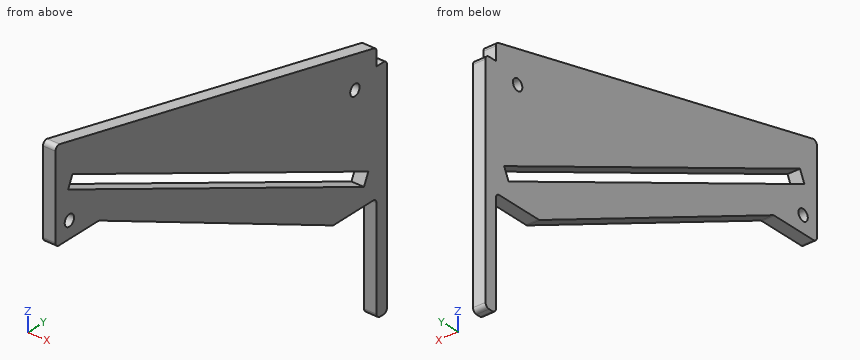
Autodesk Inventor part; units mm, degrees
ref_plane "YZ Plane" through (0, 0, 0) normal (1, 0, 0) x (0, 1, 0)
ref_plane "XZ Plane" through (0, 0, 0) normal (0, 1, 0) x (-1, 0, 0)
ref_plane "XY Plane" through (0, 0, 0) normal (0, 0, 1) x (1, 0, 0)
sketch "Sketch1" plane through (0, 0, 0) normal (1, 0, 0) x (0, 1, 0)
  line L0 (0, 0) -> (0, 25) construction
  line L1 (185, -25) -> (185, -90)
  line L2 (185, -25) -> (-25, 25) construction
  line L3 (0, 0) -> (0, 19.0476)
  line L4 (0, 19.0476) -> (185, -25)
  line L5 (0, -25) -> (0, 0)
  line L6 (185, -90) -> (160, -90)
  line L7 (0, -25) -> (25, -25)
  line L8 (25, -25) -> (160, -90)
  dimension "d0" = 25
  dimension "d1" = 65
  dimension "d2" = 185
  dimension "d10" = 25
  dimension "d11" = 25
  dimension "d17" = 25
  dimension "d20" = 25
extrude "Extrusion1" add sketch "Sketch1" along normal blind 6
sketch "Sketch3" plane through (6, 0, 0) normal (1, 0, 0) x (0, 0, -1)
  line L0 (90, 185) -> (25, 185)
  line L1 (33.1, 185) -> (141.9, 185)
  line L2 (141.9, 185) -> (141.9, 191)
  line L3 (141.9, 191) -> (33.1, 191)
  line L4 (33.1, 191) -> (33.1, 185)
  dimension "d12" = 8.1
  dimension "d14" = 6
  dimension "d21" = 108.8
extrude "Extrusion3" add sketch "Sketch3" against normal blind 6
sketch "Sketch4" plane through (6, 0, 0) normal (1, 0, 0) x (0, 0, -1)
  line L0 (0, 0) -> (85, 185) construction
  line L1 (3.34, 7.2694) -> (-2.1121, 9.7744)
  line L2 (-2.1121, 9.7744) -> (76.2079, 180.2356)
  line L3 (76.2079, 180.2356) -> (81.66, 177.7306)
  line L4 (3.34, 7.2694) -> (81.66, 177.7306)
  dimension "d23" = 185
  dimension "d24" = 85
  dimension "d28" = 8
  dimension "d29" = 8
  dimension "d32" = 6
extrude "Extrusion4" cut sketch "Sketch4" against normal through all
sketch "Sketch5" plane through (6, 0, 0) normal (1, 0, 0) x (0, 0, -1)
  line L0 (-19.0476, 0) -> (25, 0)
  line L1 (25, 0) -> (25, 25)
  line L2 (33.1, 185) -> (25, 185)
  circle A0 centre (37.5, 172.5) radius 2.7
  circle A1 centre (17, 8) radius 2.7
  point P0 (0, 0)
  dimension "d34" = 12.5
  dimension "d35" = 12.5
  dimension "d36" = 5.4
  dimension "d37" = 5.4
  dimension "d38" = 8
  dimension "d39" = 8
extrude "Extrusion5" cut sketch "Sketch5" against normal through all
fillet "Fillet1" radius 2 9 edges at (3, 185, -25) (3, 191, -33.1) (3, 191, -141.9) (3, 185, -141.9) (3, 185, -90) (3, 160, -90) (3, 25, -25) (3, 0, -25) (3, 0, 19.0476)
properties part number "ControlRightPanel"
The listing builds one solid part. Answer for the finished solid, in the listing's coordinates (mm). Coordinates: 2 decimals unless noted, no trailing zeros. Write each loop counter-clockwise with the first axis right and the second up, starting at its lowest first coordinate (ties: lowest second). Pieces come first, ordered by that corner, then holes. Notation, with made-up numbers: (8.5, -6) - (34.5, -6) arc R26 ccw to (34.5, 21) - close; hole circle Ø2 at (16.25, 64.25). An arc over 180 degrees is marked (long way). Return JSON: item names as keys, results as strings. Group by question number.
Q1. The part is cut by section C-C on y = 127.5. Write down the section's boundary in (x, z), and give its area (3 significant figures).
Q2. Flat-ended cylindrical pins translate along their axes: pin 1 Ø1.8 at (x, y) = (3.5, 18.5) entering from -Z; pin 2 Ø1 at (x, z) = (4, -90) entering from -Y; pin 3 Ø3 at (x, y) = (3, 122.5) entering from -Z; pin 4 Ø3 at (y, z) = (8, -17) entering from -X. Find the tip coordinate at first contact, or state that the pin passes through.
Q3. Find the intervals of material crossed by line 1 along Z through (x, y) = (2.2, 10); line 2 along Y through (x, z) = (5, -39) (3 decimals); line 3 along Z through (x, y) = (4.2, 172.5), in increasing order. Write a range as [from, to].
Q4. The part is cut by section D-D on z = -59. Write down the section's boundary in (x, y), and give its area (3 significant figures).
Q5. The part is cut by section B-B on z = -37.5. Write down the section's boundary in (x, y).
Q6. The part is cut by section A-A on x = 1.1. Write down the section's boundary in (y, z), and give its area (3 significant figures).
Evaluation:
{
 "1": {"outline": "(0, -74.35) - (6, -74.35) - (6, -58.58) - (0, -58.58) - close; (0, -51.98) - (6, -51.98) - (6, -11.31) - (0, -11.31) - close", "area": "339 mm2"},
 "2": {"pin 1": "stops at z = -25", "pin 2": "stops at y = 158.96", "pin 3": "stops at z = -72.67", "pin 4": "passes through"},
 "3": {"line 1": "z = [-25, -18.81], [-15.19, -4.59], [2.01, 16.67]", "line 2": "y = [54.077, 84.882], [99.254, 170.255], [174.745, 191]", "line 3": "z = [-90, -79.26], [-72.65, -40.2], [-34.8, -22.02]"},
 "4": {"outline": "(0, 95.62) - (6, 95.62) - (6, 128.41) - (0, 128.41) - close; (0, 142.78) - (6, 142.78) - (6, 191) - (0, 191) - close", "area": "486 mm2"},
 "5": {"outline": "(0, 50.96) - (6, 50.96) - (6, 81.62) - (0, 81.62) - close; (0, 95.99) - (6, 95.99) - (6, 169.8) - (0, 169.8) - close; (0, 175.2) - (6, 175.2) - (6, 191) - (0, 191) - close"},
 "6": {"outline": "(0, -23) arc R2 ccw to (2, -25) - (24.54, -25) arc R2 cw to (25.41, -25.2) - (159.59, -89.8) arc R2 ccw to (160.46, -90) - (183, -90) arc R2 cw to (185, -92) - (185, -139.9) arc R2 ccw to (187, -141.9) - (189, -141.9) arc R2 ccw to (191, -139.9) - (191, -35.1) arc R2 ccw to (189, -33.1) - (185, -33.1) - (185, -26.58) arc R2 ccw to (183.46, -24.63) - (2.46, 18.46) arc R2 ccw to (0, 16.52) - close; hole circle Ø5.4 at (8, -17); hole (7.27, -3.34) - (177.73, -81.66) - (180.24, -76.21) - (9.77, 2.11) - close; hole circle Ø5.4 at (172.5, -37.5)", "area": "9,560 mm2"}
}
